from build123d import *

# Parameters (mm, degrees)
SKETCH004_R     = 1.75
SKETCH004_W     = 11.5
SKETCH004_H     = 3
SKETCH004_W_2   = 6.5
PAD_DEPTH       = 8.5
FILLET_R        = 1
FILLET001_R     = 0.6
FILLET002_R     = 0.5
SKETCH_W        = 25.7
SKETCH_H        = 13
POCKET_DEPTH    = 3
FILLET003_R     = 0.5
SKETCH005_R     = 1.8
POCKET001_DEPTH = 2


with BuildPart() as part:
    # Sketch004 → Pad (new body)
    with BuildSketch(Plane.XZ):
        with BuildLine():
            Line((15.7, 8.35), (15.7, -0.06))
            Line((15.7, -0.06), (16.99, -0.06))
            ThreePointArc((18.99, -2.06), (18.404214, -0.645786), (16.99, -0.06))
            Line((18.99, -2.06), (18.99, -5.56))
            ThreePointArc((16.99, -7.56), (18.404214, -6.974214), (18.99, -5.56))
            Line((16.99, -7.56), (15.7, -7.56))
            Line((15.7, -8.35), (15.7, -7.56))
            ThreePointArc((14.7, -9.35), (15.407107, -9.057107), (15.7, -8.35))
            Line((14.7, -9.35), (12, -9.35))
            Line((12, -7.41), (12, -9.35))
            Line((-12, -7.41), (12, -7.41))
            Line((-12, -7.41), (-12, -9.35))
            Line((-12, -9.35), (-13.7, -9.35))
            ThreePointArc((-14.7, -8.35), (-14.407107, -9.057107), (-13.7, -9.35))
            Line((-14.7, -8.35), (-14.7, 10.64))
            ThreePointArc((-12.7, 12.64), (-14.114214, 12.054214), (-14.7, 10.64))
            Line((-12.7, 12.64), (-8.41, 12.64))
            ThreePointArc((-6.41, 10.64), (-6.995786, 12.054214), (-8.41, 12.64))
            Line((-6.41, 10.64), (-6.41, 9.35))
            Line((-6.41, 9.35), (14.7, 9.35))
            ThreePointArc((15.7, 8.35), (15.407107, 9.057107), (14.7, 9.35))
        make_face()
        with Locations((-10.16, 8.89)):
            Circle(SKETCH004_R, mode=Mode.SUBTRACT)
        with Locations((15.24, -3.81)):
            Circle(SKETCH004_R, mode=Mode.SUBTRACT)
        with Locations((-6.35, -3.81)):
            Rectangle(SKETCH004_W, SKETCH004_H, mode=Mode.SUBTRACT)
        with Locations((8.91, -3.81)):
            Rectangle(SKETCH004_W_2, SKETCH004_H, mode=Mode.SUBTRACT)
    extrude(amount=-PAD_DEPTH)

    # Fillet
    fillet_edges = [part.edges().sort_by_distance(p)[0] for p in [
        (12.16, 4.25, -5.31),
        (5.66, 4.25, -2.31),
        (12.16, 4.25, -2.31),
        (5.66, 4.25, -5.31),
        (-0.6, 4.25, -2.31),
        (-12.1, 4.25, -2.31),
        (-0.6, 4.25, -5.31),
        (-12.1, 4.25, -5.31),
    ]]
    fillet(fillet_edges, radius=FILLET_R)

    # Fillet001
    fillet001_edges = [part.edges().sort_by_distance(p)[0] for p in [
        (-6.41, 4.25, 9.35),
        (15.7, 4.25, -0.06),
    ]]
    fillet(fillet001_edges, radius=FILLET001_R)

    # Fillet002
    fillet002_edges = [part.edges().sort_by_distance(p)[0] for p in [
        (12, 4.25, -9.35),
        (-12, 4.25, -9.35),
        (-12, 4.25, -7.41),
        (12, 4.25, -7.41),
    ]]
    fillet(fillet002_edges, radius=FILLET002_R)

    # Sketch (on Face1 of Fillet002) → Pocket (cut)
    with BuildSketch(Plane.XZ):
        Rectangle(SKETCH_W, SKETCH_H)
    extrude(amount=-POCKET_DEPTH, mode=Mode.SUBTRACT)

    # Fillet003
    fillet003_edges = [part.edges().sort_by_distance(p)[0] for p in [
        (-12.85, 1.5, 6.5),
        (12.85, 1.5, 6.5),
        (-12.85, 1.5, -6.5),
        (12.85, 1.5, -6.5),
    ]]
    fillet(fillet003_edges, radius=FILLET003_R)

    # Sketch005 (on Face39 of Fillet003) → Pocket001 (cut)
    with BuildSketch(Plane.XZ.offset(-3)):
        Circle(SKETCH005_R)
        with BuildLine():
            Line((-12.85, 1.5), (-3.5, 1.5))
            ThreePointArc((-3.5, 1.5), (-2.085786, 2.085786), (-1.5, 3.5))
            Line((-1.5, 3.5), (-1.5, 6.5))
            Line((-1.5, 6.5), (-12.35, 6.5))
            ThreePointArc((-12.35, 6.5), (-12.703553, 6.353553), (-12.85, 6))
            Line((-12.85, 6), (-12.85, 1.5))
        make_face()
        with BuildLine():
            Line((1.5, 6.5), (12.35, 6.5))
            ThreePointArc((12.85, 6), (12.703553, 6.353553), (12.35, 6.5))
            Line((12.85, 6), (12.85, 1.5))
            Line((12.85, 1.5), (3.5, 1.5))
            ThreePointArc((1.5, 3.5), (2.085786, 2.085786), (3.5, 1.5))
            Line((1.5, 3.5), (1.5, 6.5))
        make_face()
        with BuildLine():
            Line((12.85, -1.5), (3.5, -1.5))
            ThreePointArc((3.5, -1.5), (2.085786, -2.085786), (1.5, -3.5))
            Line((1.5, -3.5), (1.5, -6.5))
            Line((1.5, -6.5), (12.35, -6.5))
            ThreePointArc((12.35, -6.5), (12.703553, -6.353553), (12.85, -6))
            Line((12.85, -6), (12.85, -1.5))
        make_face()
        with BuildLine():
            Line((-12.85, -1.5), (-3.5, -1.5))
            ThreePointArc((-1.5, -3.5), (-2.085786, -2.085786), (-3.5, -1.5))
            Line((-1.5, -3.5), (-1.5, -6.5))
            Line((-1.5, -6.5), (-12.35, -6.5))
            ThreePointArc((-12.85, -6), (-12.703553, -6.353553), (-12.35, -6.5))
            Line((-12.85, -6), (-12.85, -1.5))
        make_face()
    extrude(amount=-POCKET001_DEPTH, mode=Mode.SUBTRACT)


solid = part.part
Can you work these out from the model? Positions are in its coordinate system, mm. A direction names the side the tool comes from. Coordinates: 2 decimals unless noted, no trailing zeros. Loops run counter-clockwise (first coordinate to the right, second up) from the corner with the lowest first, then second, coordinate; pieces in that order, holes last. Notation, with made-up numbers: (28, 39) - (60, 39) arc R15 cw to (60, 67) - close; hole circle Ø8 at (-14, -10.75). An arc over 180 degrees is marked (long way). Put each result on its own line as item: value. Start each with the question number.
Item 1: For pin 1 (5.5 mm diameter, centred on x = 15.24, z = -3.81, fed in from -Y); pin 2 (1.5 mm diameter, centred on x = -1, y = 7, fed in from +Z); pin 3 (5 mm diameter, centred on y = 7.5, z = 3, fed in from +X); pin 4 (4 mm diameter, centred on x = 2.5, y = 3.5, fed in from -Z), each with a flat end and sliding along its axis, tell me the tip position at first contact or that it passes through.
Item 2: Suppose I cut it at B-B (z = 8). Please give me the cut outline in (x, y), and give its area (3 significant figures).
Item 3: Suppose I cut it at D-D (y = 7.25). State how many separate pieces and enclosed holes the cut face has, and give its area (3 significant figures).
Item 4: If I drill on line 1 along Z through (x, y) = (-10.16, 2.75); line 2 along X through (y, z) = (6.75, -3.75); line 3 along Z through (x, y) = (9, 1), over which ranges is the centre line in solid material (lowest first)?
Item 5: Suppose I cut it at A-A (x = -10.16). Please give me the cut outline in (y, z), and give its area (3 significant figures).
Item 6: Which directions (+Z, -Z, +X, -X, +Y, -Y) give clear straight access to the entire face, cutting with the end or side of a thin tool? Please do faces 4 (the face through (5.945, 6.774, -2.611)), 5 (the face through (2.07, 3.99, 2.1)), 6 (the face through (12, 4.2, -8.4)).
Item 7: Suppose I cut it at C-C (x = 6). Please give me the cut outline in (y, z), and give its area (3 significant figures).
Item 8: If we mould it in two halves opening along X, with no side actions, what happens to faces 1 (the face through (0, 2, -6.5)), 2 (the face through (4, 4, 9.35)), 3 (the face through (-6.98, 4.19, 12.04))? For each: +X half, -X half, draft (parallel to the pull), parting line (faces both ways), or undercut.
Here are the results:
1. pin 1: y = 0
1. pin 2: z = 9.35
1. pin 3: x = 15.7
1. pin 4: z = -7.41
2. outline: (-14.7, 0) - (-11.67, 0) - (-11.67, 8.5) - (-14.7, 8.5) - close; (-8.65, 0) - (15.7, 0) - (15.7, 8.5) - (-8.65, 8.5) - close
2. area: 233 mm²
3. separate pieces: 1
3. enclosed holes: 4
3. area: 498 mm²
4. line 1: -7.41 to -6.5, 6.5 to 7.14, 10.64 to 12.64
4. line 2: -14.7 to -12.1, -0.6 to 5.66, 12.16 to 13.49, 16.99 to 18.99
4. line 3: -7.41 to -6.5, 6.5 to 9.35
5. outline: (0, -7.41) - (8.5, -7.41) - (8.5, -5.31) - (5, -5.31) - (5, -6.5) - (0, -6.5) - close; (0, 6.5) - (5, 6.5) - (5, 1.5) - (3, 1.5) - (3, -1.5) - (5, -1.5) - (5, -2.31) - (8.5, -2.31) - (8.5, 7.14) - (0, 7.14) - close; (0, 10.64) - (8.5, 10.64) - (8.5, 12.64) - (0, 12.64) - close
5. area: 71.2 mm²
6. face 4: +Y, -Y
6. face 5: -Y
6. face 6: -Z, +Y, -Y
7. outline: (0, -7.41) - (8.5, -7.41) - (8.5, -5.06) - (5, -5.06) - (5, -6.5) - (0, -6.5) - close; (0, 6.5) - (5, 6.5) - (5, 1.5) - (3, 1.5) - (3, -1.5) - (5, -1.5) - (5, -2.56) - (8.5, -2.56) - (8.5, 9.35) - (0, 9.35) - close
7. area: 74.7 mm²
8. face 1: undercut
8. face 2: draft
8. face 3: +X half
